Could you check a few things on this model? Use its own coordinates, in mm. Give positions to 0.01 mm unless a question says otherwise; leave off trailing zeros. Loops run counter-clockwise (first coordinate to the right, second up) from the corner with the lowest first, then second, coordinate; pieces in that order, holes last.
1. Imagine slicing it at B-B (z = 3). List the corners of the cut face in (x, y) for me.
2. Imagine slicing it at C-C (x = 0). List the corners of the cut face in (y, z) for me.
3. I need wall thicknesses on line 1 along Y through (x, z) = (0, 7); line 2 along Y through (x, z) = (5, 5.75); line 3 along Y through (x, z) = (-6, 6.75). Which ranges of each line are inside material? Lowest first, please.
4. For P1, Ø4.5, axis at x = 35.33, y = 42.48, coming from the -Z side; P2, Ø4, axis at x = -18.5, z = 6.5, coming from the -Y side; P3, Ø5, axis at x = -35.33, y = 42.48, coming from the +Z side; P4, Ø1, axis at y = 10.5, z = 7.5, coming from the +X side, each with a flat end and sliding along its axis, tell me the tip position at first contact or that it passes through.
5. Imagine slicing it at A-A (x = 18). List the corners of the cut face in (y, z) for me.
6. Imagine slicing it at D-D (y = 35.5). List the corners of the cut face in (x, z) for me.
7. Thinking about a two-plate mould opening in Y: for faces 1 (the flat face through (1, 50.5, 5)), 2 (the conical face through (36.472, 44.277, 8.125)), 3 (the flat face through (-1, 29, 0)), which applies, +Y half, -Y half, draft (parallel to the pull), parting line (faces both ways), or undercut?
```python
from build123d import *

# Parameters (mm, degrees)
F0_R     = 20.5
F0_R_2   = 2
F1_DEPTH = 10
F2_SIZE  = 2
F3_R     = 5


with BuildPart() as f1:
    # F0 (on Top) → F1 (new body)
    with BuildSketch(Plane.XY):
        with BuildLine():
            Line((-50, 50.5), (-30.5, 0))
            ThreePointArc((-30.5, 0), (0, -30.5), (30.5, 0))
            Line((30.5, 0), (50, 50.5))
            Line((50, 50.5), (-50, 50.5))
        make_face()
        Circle(F0_R, mode=Mode.SUBTRACT)
        with Locations((-35.330024, 42.484712)):
            Circle(F0_R_2, mode=Mode.SUBTRACT)
        with Locations((0, 35.5)):
            Circle(F0_R_2, mode=Mode.SUBTRACT)
        with Locations((35.330024, 42.484712)):
            Circle(F0_R_2, mode=Mode.SUBTRACT)
    extrude(amount=F1_DEPTH)

    # F2
    f2_edges = [f1.edges().sort_by_distance(p)[0] for p in [
        (-37.330024, 42.484712, 10),
        (-2, 35.5, 10),
        (33.330024, 42.484712, 10),
    ]]
    chamfer(f2_edges, length=F2_SIZE)

    # F3
    f3_edges = [f1.edges().sort_by_distance(p)[0] for p in [
        (50, 50.5, 5),
        (-50, 50.5, 5),
    ]]
    fillet(f3_edges, radius=F3_R)


solid = f1.part
```
Derived:
1. outline: (-47.37, 43.7) - (-30.5, 0) arc R30.5 ccw to (30.5, 0) - (47.37, 43.7) arc R5 ccw to (42.71, 50.5) - (-42.71, 50.5) arc R5 ccw to start; hole circle Ø4 at (-35.33, 42.48); hole circle Ø41 at (0, 0); hole circle Ø4 at (0, 35.5); hole circle Ø4 at (35.33, 42.48)
2. outline: (-30.5, 0) - (-20.5, 0) - (-20.5, 10) - (-30.5, 10) - close; (20.5, 0) - (33.5, 0) - (33.5, 8) - (31.5, 10) - (20.5, 10) - close; (37.5, 0) - (50.5, 0) - (50.5, 10) - (39.5, 10) - (37.5, 8) - close
3. line 1: y = -30.5 to -20.5, 20.5 to 33.5, 37.5 to 50.5
3. line 2: y = -30.09 to -19.88, 19.88 to 50.5
3. line 3: y = -29.9 to -19.6, 19.6 to 50.5
4. P1: stops at z = 0
4. P2: stops at y = -25.65
4. P3: stops at z = 8.5
4. P4: stops at x = 34.75
5. outline: (-24.62, 0) - (-9.81, 0) - (-9.81, 10) - (-24.62, 10) - close; (9.81, 0) - (50.5, 0) - (50.5, 10) - (9.81, 10) - close
6. outline: (-44.21, 0) - (-2, 0) - (-2, 8) - (-4, 10) - (-44.21, 10) - close; (2, 0) - (44.21, 0) - (44.21, 10) - (4, 10) - (2, 8) - close
7. face 1: +Y half
7. face 2: undercut
7. face 3: draft
